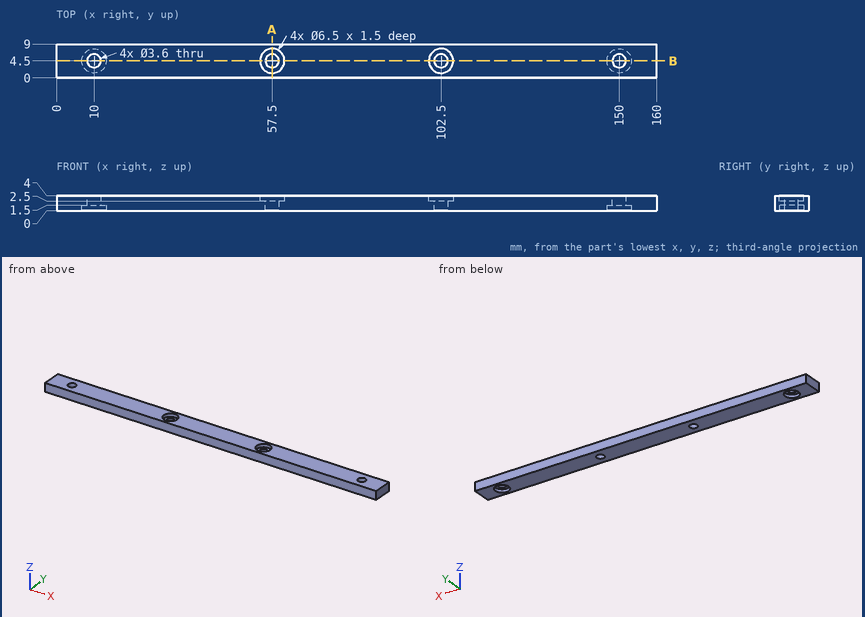
Here's the drawing with two shaded views (mm, measured from the low corner). I have some questions. Give positions to 0.01 mm unless a question says otherwise; leave off trailing zeros. Order: outer loops, then holes, each group sorted by start corner. A loop starts at its lowest first (then second) coordinate and runs counter-clockwise, first axis right, second up. Notation, with made-up numbers: (0, 50) - (5, 50) arc R32 cw to (5, 83) - close; hole circle Ø4 at (26, 80). An arc over 180 degrees is marked (long way). Use a Markdown table: item, result. Add a question column.
Q1. Please list where these lines run through material, in increasing order: line 1 along X through (y, z) = (4.75, 2.6); line 2 along Y through (x, z) = (10, 0.8); line 3 along X through (y, z) = (4, 2.9).
Q2. If we section it at A-A on x = 57.5: Write out the boundary of the cut face in (y, z).
Q3. If we section it at B-B on y = 4.5: Count the separate pieces of the cut face and the enclosed holes in it, plus the area to 3 significant figures.
Q4. I'm going to push flat-ended pins straight in: pin 1 (2 mm diameter, centred on x = 149.5, y = 6, fed in from -Z); pin 2 (3 mm diameter, centred on x = 58.5, y = 4.5, fed in from +Z). Where does each tip first touch, or does it pass through?
Answers follow:
| question | item | result |
|---|---|---|
| 1 | line 1 | x = 0 to 8.22, 11.78 to 54.26, 60.74 to 99.26, 105.74 to 148.22, 151.78 to 160 |
| 1 | line 2 | y = 0 to 1.25, 7.75 to 9 |
| 1 | line 3 | x = 0 to 8.27, 11.73 to 54.29, 60.71 to 99.29, 105.71 to 148.27, 151.73 to 160 |
| 2 | outline | (0, 0) - (2.7, 0) - (2.7, 2.5) - (1.25, 2.5) - (1.25, 4) - (0, 4) - close; (6.3, 0) - (9, 0) - (9, 4) - (7.75, 4) - (7.75, 2.5) - (6.3, 2.5) - close |
| 3 | separate pieces | 5 |
| 3 | enclosed holes | 0 |
| 3 | area | 565 mm^2 |
| 4 | pin 1 | stops at z = 1.5 |
| 4 | pin 2 | stops at z = 2.5 |
